Geometry check sheet. Reference: drawing and pictorial views, mm from the part's lowest x, y, z. A direction names the side the tool comes from. Coordinates: 2 decimals unless noted, no trailing zeros. Write each loop counter-clockwise with the first axis right and the second up, starting at its lowest first coordinate (ties: lowest second). Pieces come first, ordered by that corner, then holes. Notation, with made-up numbers: (75, -11.75) -> (128, -11.75) arc R7 cw to (128, -1.75) -> close; hole circle Ø9 at (-8.5, 8.5). An arc over 180 degrees is marked (long way). Use a Markdown table: item, result.
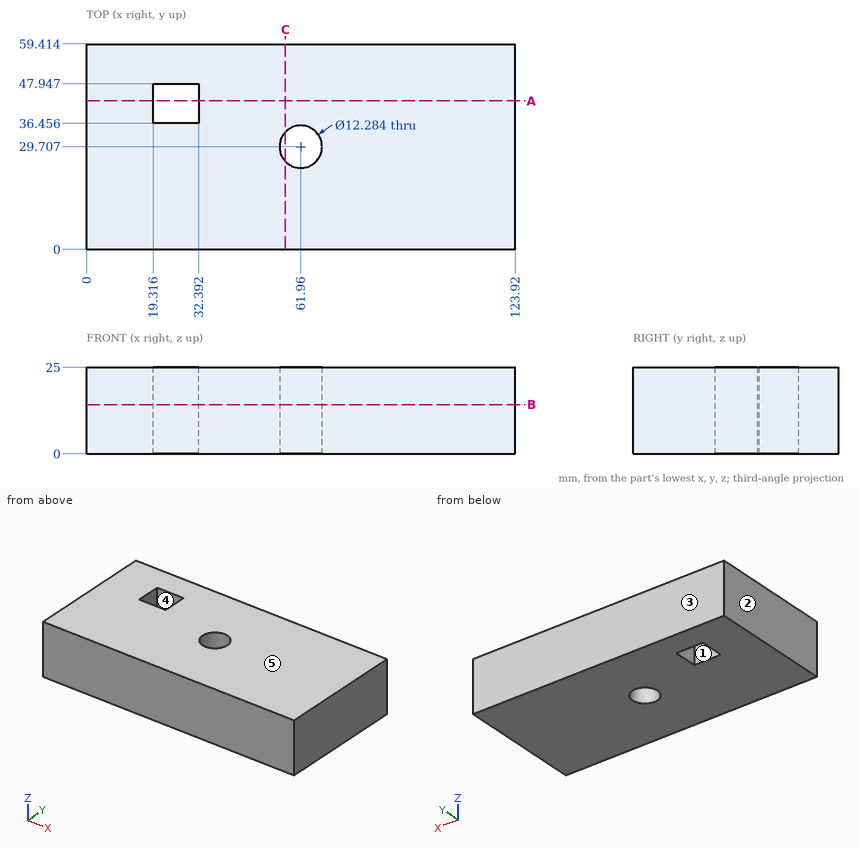
Item 1: Section check A-A on y = 43. Record the boundary of the cut face in (x, z), then the cut area to 3 significant figures.
Answer block:
| item | result |
|---|---|
| outline | (0, 0) -> (19.32, 0) -> (19.32, 25) -> (0, 25) -> close; (32.39, 0) -> (123.92, 0) -> (123.92, 25) -> (32.39, 25) -> close |
| area | 2,770 mm^2 |
Item 2: Mould release check, pull along Y, two halves, no side actions. Record for the marked faces 1, 2 and 3: +Y half, -Y half, draft (parallel to the pull), parting line (faces both ways), or undercut.
Answer block:
| item | result |
|---|---|
| face 1 | undercut |
| face 2 | draft |
| face 3 | +Y half |
Item 3: Thickness scan on L1, parallel to X at y = 38, z = 19.25; L2, parallel to X at y = 28, z = 11; L3, parallel to Y at x = 63.5, z = 20.75 (1 decimal). Record the ranges inside material, lowest first. Write a range as [from, to].
Answer block:
| item | result |
|---|---|
| L1 | x = [0, 19.32], [32.39, 123.92] |
| L2 | x = [0, 56.06], [67.86, 123.92] |
| L3 | y = [0, 23.8], [35.7, 59.4] |
Item 4: Tool access check on the marked faces 4 and 5. Record the directions out of +Z, -Z, +X, -X, +Y, -Y that give a thin tool (end or side, any length) a straight path to the whole face; none if there is none.
Answer block:
| item | result |
|---|---|
| face 4 | +Z, -Z |
| face 5 | +Z, +X, -X, +Y, -Y |
Item 5: Section check B-B on z = 14.25. Record the boundary of the cut face in (x, y) (1 decimal), then the cut area to 3 significant figures.
Answer block:
| item | result |
|---|---|
| outline | (0, 0) -> (123.9, 0) -> (123.9, 59.4) -> (0, 59.4) -> close; hole (19.3, 36.5) -> (32.4, 36.5) -> (32.4, 47.9) -> (19.3, 47.9) -> close; hole circle Ø12.3 at (62, 29.7) |
| area | 7,090 mm^2 |
Item 6: Section check C-C on x = 57.5. Record the boundary of the cut face in (y, z) (1 decimal).
Answer block:
| item | result |
|---|---|
| outline | (0, 0) -> (25.5, 0) -> (25.5, 25) -> (0, 25) -> close; (33.9, 0) -> (59.4, 0) -> (59.4, 25) -> (33.9, 25) -> close |
